Could you check a few things on this model? Use its own coordinates, in mm. Face numbers are marked on the shaded views. A direction names the side the tool comes from. Coordinates: 2 decimals unless noted, no trailing zeros. Write each loop counter-clockwise with the first axis right and the second up, starting at its lowest first coordinate (ties: lowest second). Pieces come first, ordered by that corner, then holes. Notation, with made-up numbers: (25.5, 87) - (84.5, 87) arc R14 ccw to (84.5, 113) - close; hole circle Ø3 at (46, 86). An arc over 180 degrees is marked (long way). Write item = value, one per line. Start each with the question number.
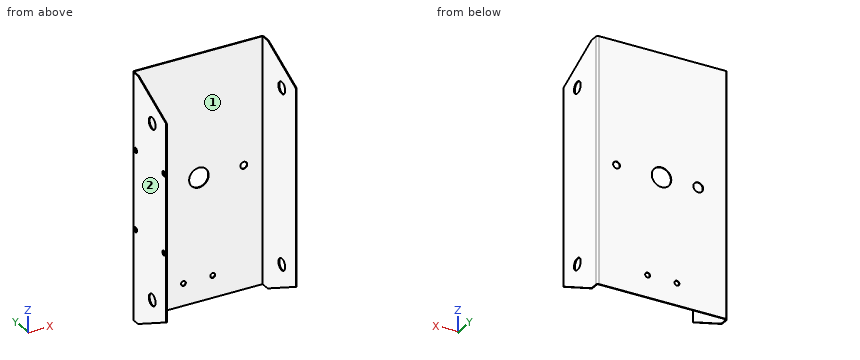
```python
from build123d import *

# Parameters (mm, degrees)
BOSS_EXTRUDE1_DEPTH     = 250
CUT_EXTRUDE1_DEPTH      = 250
CUT_EXTRUDE2_DEPTH      = 290.7486918
CUT_EXTRUDE2_DEPTH_BACK = 290.7486918
SKETCH3_R               = 6
FILLET1_R               = 2
SKETCH5_R               = 10
CUT_EXTRUDE3_DEPTH      = 10
SKETCH6_R               = 2.5
CUT_EXTRUDE4_DEPTH      = 10
SKETCH7_R               = 3.5
SKETCH7_R_2             = 5
CUT_EXTRUDE5_DEPTH      = 10
SKETCH9_R               = 2.5
CUT_EXTRUDE8_DEPTH      = 14


with BuildPart() as part:
    # Sketch1 → Boss-Extrude1 (new body)
    with BuildSketch(Plane.XY):
        Polygon((-66.81, -60), (-66.81, 0), (66.81, 0), (66.81, -60), (65.93, -60), (65.93, -0.75), (-65.93, -0.75), (-65.93, -60), align=None)
    extrude(amount=BOSS_EXTRUDE1_DEPTH)

    # Sketch2 → Cut-Extrude1 (cut)
    with BuildSketch(Plane(origin=(66.81, 0, 0), x_dir=(0, 0, -1), z_dir=(1, 0, 0))):
        Polygon((-225, -60), (-250, -10), (-250, -60), align=None)
        Polygon((0, -10), (-25, -60), (0, -60), align=None)
    extrude(amount=-CUT_EXTRUDE1_DEPTH, mode=Mode.SUBTRACT)

    # Sketch3 → Cut-Extrude2 (cut, two sides: drawn at the far end of the back side and taken through both)
    with BuildSketch(Plane(origin=(66.81, 0, 0), x_dir=(0, 0, -1), z_dir=(1, 0, 0)).offset(-CUT_EXTRUDE2_DEPTH_BACK)):
        with Locations(Location((-214, -35, 0), (0, 0, 90))):
            Circle(SKETCH3_R)
        with Locations(Location((-36, -35, 0), (0, 0, 90))):
            Circle(SKETCH3_R)
    extrude(amount=CUT_EXTRUDE2_DEPTH + CUT_EXTRUDE2_DEPTH_BACK, mode=Mode.SUBTRACT)

    # Fillet1
    fillet1_edges = [part.edges().sort_by_distance(p)[0] for p in [
        (-66.81, 0, 125),
        (66.81, 0, 125),
    ]]
    fillet(fillet1_edges, radius=FILLET1_R)

    # Sketch5 → Cut-Extrude3 (cut)
    with BuildSketch(Plane(origin=(0, 0, 0), x_dir=(1, 0, 0), z_dir=(0, 1, 0))):
        with Locations(Location((0.81, -125, 0), (0, 0, 180))):
            Circle(SKETCH5_R)
    extrude(amount=-CUT_EXTRUDE3_DEPTH, mode=Mode.SUBTRACT)

    # Sketch6 → Cut-Extrude4 (cut)
    with BuildSketch(Plane(origin=(-65.93, 0, 0), x_dir=(0, 0, -1), z_dir=(1, 0, 0))):
        with Locations(Location((-173, -55.7, 0), (0, 0, 90))):
            Circle(SKETCH6_R)
        with Locations(Location((-93, -55.7, 0), (0, 0, 90))):
            Circle(SKETCH6_R)
        with Locations(Location((-93, -5.7, 0), (0, 0, 90))):
            Circle(SKETCH6_R)
        with Locations(Location((-173, -5.7, 0), (0, 0, 90))):
            Circle(SKETCH6_R)
    extrude(amount=-CUT_EXTRUDE4_DEPTH, mode=Mode.SUBTRACT)

    # Sketch7 → Cut-Extrude5 (cut)
    with BuildSketch(Plane(origin=(0, 0, 0), x_dir=(1, 0, 0), z_dir=(0, 1, 0))):
        with Locations(Location((46.81, -125, 0), (0, 0, 180))):
            Circle(SKETCH7_R)
        with Locations(Location((-36.81, -125, 0), (0, 0, 180))):
            Circle(SKETCH7_R_2)
    extrude(amount=-CUT_EXTRUDE5_DEPTH, mode=Mode.SUBTRACT)

    # Sketch9 → Cut-Extrude8 (cut)
    with BuildSketch(Plane(origin=(0, 0, 0), x_dir=(1, 0, 0), z_dir=(0, 1, 0))):
        with Locations(Location((-15, -22.5, 0), (0, 0, 180))):
            Circle(SKETCH9_R)
        with Locations(Location((15, -22.5, 0), (0, 0, 180))):
            Circle(SKETCH9_R)
    extrude(amount=-CUT_EXTRUDE8_DEPTH, mode=Mode.SUBTRACT)


solid = part.part
```
1) For P1, Ø9, axis at x = 46.81, z = 125, coming from the -Y side; P2, Ø3, axis at y = -55.7, z = 173, coming from the -X side, each with a flat end and sliding along its axis, tell me the tip position at first contact or that it passes through.
2) Which directions (+Z, -Z, +X, -X, +Y, -Y) give clear straight access to the entire face, cutting with the end or side of a thin tool? Please do the marked faces 1 and 2.
3) If I drill on probe 1 along Z at (x, y) = (-36.81, -0.5); probe 2 along X at (y, z) = (-8.5, 91); probe 3 along Z at (x, y) = (-66.55, -35), over which ranges is the centre line in solid material (lowest first)? Write a range as [from, to].
4) Suppose I cut it at C-C on z = 125. Please give me the cut outline in (x, y).
5) Suppose I cut it at B-B on y = -5.7. Please give me the cut outline in (x, z).
6) Suppose I cut it at D-D on x = 46.81. Please give me the cut outline in (y, z).
7) Suppose I cut it at A-A on z = 36. Please give me the cut outline in (x, y), plus the area to 3 significant figures.
Reply:
q1.P1 = -0.75
q1.P2 = 65.93
q2.face_1 = +Z, -Z, -Y
q2.face_2 = +Z, -Z, -X, +Y, -Y
q3.probe_1 = [0, 120], [130, 250]
q3.probe_2 = [-66.81, -65.93], [65.93, 66.81]
q3.probe_3 = [12.5, 30], [42, 208], [220, 237.5]
q4.outline = (-66.81, -60) - (-65.93, -60) - (-65.93, -0.75) - (-41.81, -0.75) - (-41.81, 0) - (-64.81, 0) arc R2 ccw to (-66.81, -2) - close; (-31.81, -0.75) - (-9.19, -0.75) - (-9.19, 0) - (-31.81, 0) - close; (10.81, -0.75) - (43.31, -0.75) - (43.31, 0) - (10.81, 0) - close; (50.31, -0.75) - (65.93, -0.75) - (65.93, -60) - (66.81, -60) - (66.81, -2) arc R2 ccw to (64.81, 0) - (50.31, 0) - close
q5.outline = (-66.81, 0) - (-65.93, 0) - (-65.93, 90.5) - (-66.81, 90.5) - close; (-66.81, 95.5) - (-65.93, 95.5) - (-65.93, 170.5) - (-66.81, 170.5) - close; (-66.81, 175.5) - (-65.93, 175.5) - (-65.93, 250) - (-66.81, 250) - close; (65.93, 0) - (66.81, 0) - (66.81, 250) - (65.93, 250) - close
q6.outline = (-0.75, 0) - (0, 0) - (0, 121.5) - (-0.75, 121.5) - close; (-0.75, 128.5) - (0, 128.5) - (0, 250) - (-0.75, 250) - close
q7.outline = (-66.81, -60) - (-65.93, -60) - (-65.93, -41) - (-66.81, -41) - close; (-66.81, -29) - (-65.93, -29) - (-65.93, -0.75) - (65.93, -0.75) - (65.93, -29) - (66.81, -29) - (66.81, -2) arc R2 ccw to (64.81, 0) - (-64.81, 0) arc R2 ccw to (-66.81, -2) - close; (65.93, -60) - (66.81, -60) - (66.81, -41) - (65.93, -41) - close
q7.area = 182 mm^2
